```python
from build123d import *

# Parameters (mm, degrees)
SKETCH1_R           = 14.55
BOSS_EXTRUDE1_DEPTH = 9.85
SKETCH3_R           = 14.55
BOSS_EXTRUDE3_DEPTH = 2.85
BOSS_EXTRUDE3_TAPER = 25
SKETCH4_R           = 10.875
BOSS_EXTRUDE4_DEPTH = 13.3
SKETCH2_W           = 31
SKETCH2_H           = 40
BOSS_EXTRUDE2_DEPTH = 37


with BuildPart() as part:
    # Sketch1 → Boss-Extrude1 (new body)
    with BuildSketch(Plane.XY):
        Circle(SKETCH1_R)
    extrude(amount=BOSS_EXTRUDE1_DEPTH)

    # Sketch3 → Boss-Extrude3 (add)
    with BuildSketch(Plane.XY.offset(9.85)):
        Circle(SKETCH3_R)
    extrude(amount=BOSS_EXTRUDE3_DEPTH, taper=BOSS_EXTRUDE3_TAPER)

    # Sketch4 → Boss-Extrude4 (add)
    with BuildSketch(Plane.XY):
        Circle(SKETCH4_R)
    extrude(amount=-BOSS_EXTRUDE4_DEPTH)

    # Sketch2 → Boss-Extrude2 (add)
    with BuildSketch(Plane.XY.offset(-13.3)):
        Rectangle(SKETCH2_W, SKETCH2_H)
    extrude(amount=-BOSS_EXTRUDE2_DEPTH)


solid = part.part
```
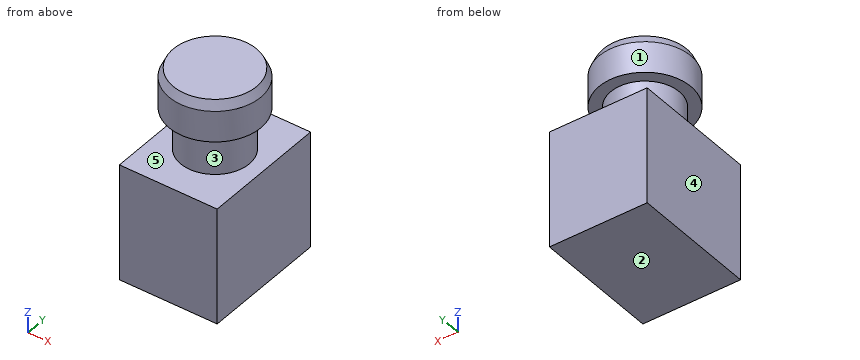
The model under review builds one solid part; all positions refer to its coordinate system, in mm. Face numbers are marked on the shaded views. A direction names the side the tool comes from. Round coordinates to 2 decimals unless told otherwise and drop trailing zeros. Loops run counter-clockwise (first coordinate to the right, second up) from the corner with the lowest first, then second, coordinate; pieces in that order, holes last. Notation, with made-up numbers: (77.25, -7) - (133.25, -7) arc R16 ccw to (133.25, 17) - close; hole circle Ø1 at (53, 44). An arc over 180 degrees is marked (long way). Use a Markdown table: item, result. Add a question column.
Q1. Add section B-B (y = 0). State the section outline as (x, z) points (3 decimals).
Q2. For probe 1 along Z at (x, y) = (12, -2.5); probe 2 along Z at (x, y) = (-12.5, 7.5); probe 3 along Y at (x, z) = (-3.5, -6.5), list the stretches that pass through material, from the lowest coordinate up.
Q3. Add section C-C (z = -5). State the section outline as (x, y) points (3 decimals), plus the area to 3 significant figures.
Q4. Add section A-A (x = 0). State the section outline as (y, z) points (3 decimals), plus the area to 3 significant figures.
Q5. Machinability: for the marked faces 4 and 5, which of the approach directions +Z, -Z, +X, -X, +Y, -Y give a long, thin tool a straight path to every point of the face, cutting with its end or side? Answer none if there is none.
Q6. Insertion check: pin 1 Ø1.5 at (y, z) = (-6, -6.5) entering from -X; pin 2 Ø5 at (x, z) = (-11.5, -5) entering from +Y. Each pin has a flat end and moves straight along its axis. Give the tip position at first contact, or say it passes through.
Q7. Add section D-D (y = -16). State the section outline as (x, z) points.
Q8. The part is to be moulded in two halves that separate along Z. For the marked faces 1, 2 and 3, say which applies: pulls with the +Z half, pulls with the -Z half, needs draft (parallel to the pull), parting line crosses it, or undercut.
Worked answers:
| question | item | result |
|---|---|---|
| 1 | outline | (-15.5, -50.3) - (15.5, -50.3) - (15.5, -13.3) - (10.875, -13.3) - (10.875, 0) - (14.55, 0) - (14.55, 9.85) - (13.221, 12.7) - (-13.221, 12.7) - (-14.55, 9.85) - (-14.55, 0) - (-10.875, 0) - (-10.875, -13.3) - (-15.5, -13.3) - close |
| 2 | probe 1 | -50.3 to -13.3, 0 to 12.7 |
| 2 | probe 2 | -50.3 to -13.3 |
| 2 | probe 3 | -10.3 to 10.3 |
| 3 | outline | circle Ø21.75 at (0, 0) |
| 3 | area | 372 mm² |
| 4 | outline | (-20, -50.3) - (20, -50.3) - (20, -13.3) - (10.875, -13.3) - (10.875, 0) - (14.55, 0) - (14.55, 9.85) - (13.221, 12.7) - (-13.221, 12.7) - (-14.55, 9.85) - (-14.55, 0) - (-10.875, 0) - (-10.875, -13.3) - (-20, -13.3) - close |
| 4 | area | 2,140 mm² |
| 5 | face 4 | +Z, -Z, -X, +Y, -Y |
| 5 | face 5 | none |
| 6 | pin 1 | x = -9.52 |
| 6 | pin 2 | y = 6.1 |
| 7 | outline | (-15.5, -50.3) - (15.5, -50.3) - (15.5, -13.3) - (-15.5, -13.3) - close |
| 8 | face 1 | needs draft |
| 8 | face 2 | pulls with the -Z half |
| 8 | face 3 | undercut |
